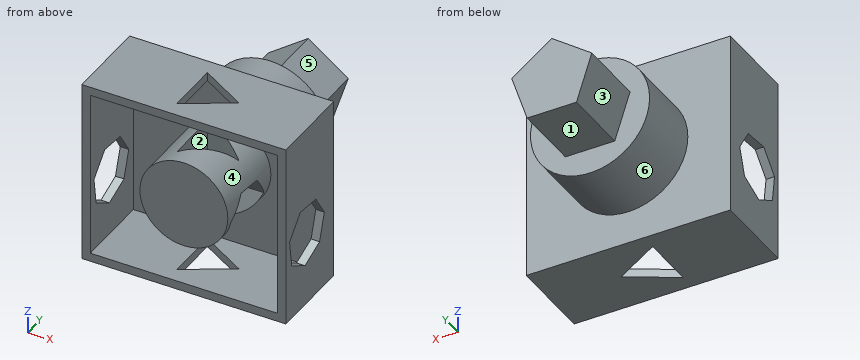
```python
from build123d import *

# Parameters (mm, degrees)
F0_W      = 76.2
F0_H      = 68.939676
F10_DEPTH = 31.75
F1_T      = -3.175
F2_R      = 22.225
F3_DEPTH  = 25.4
F5_DEPTH  = 25.4
F11_R     = 16.418379
F6_DEPTH  = 28.575
F8_DEPTH  = 76.201
F12_DEPTH = 68.940675


with BuildPart() as f10:
    # F0 (on Front) → F10 (new body)
    with BuildSketch(Plane.XZ):
        Rectangle(F0_W, F0_H)
    extrude(amount=F10_DEPTH)

    # F1
    f1_openings = [f10.faces().sort_by_distance(p)[0] for p in [
        (0, -31.75, 0),
    ]]
    offset(amount=F1_T, openings=f1_openings)

    # F2 (on face) → F3 (join)
    with BuildSketch(Plane(origin=(0, 0, 0), x_dir=(-1, 0, 0), z_dir=(0, 1, 0))):
        Circle(F2_R)
    extrude(amount=F3_DEPTH)

    # F4 (on face) → F5 (join)
    with BuildSketch(Plane(origin=(0, 25.4, 0), x_dir=(-1, 0, 0), z_dir=(0, 1, 0))):
        Polygon((-9.22709, -12.7), (9.22709, -12.7), (14.929745, 4.850968), (0, 15.698063), (-14.929745, 4.850968), align=None)
    extrude(amount=F5_DEPTH)

    # F11 (on face) → F6 (join, through all)
    with BuildSketch(Plane.XZ.offset(3.175)):
        Circle(F11_R)
    extrude(amount=F6_DEPTH)

    # F7 (on face) → F8 (cut, through all)
    with BuildSketch(Plane.YZ.offset(38.1)):
        Polygon((-27.926964, -13.740439), (-19.06612, -19.032735), (-9.40379, -15.40474), (-6.215907, -5.588409), (-11.903011, 3.024361), (-22.182597, 3.947978), (-29.313927, -3.51306), align=None)
    extrude(amount=-F8_DEPTH, mode=Mode.SUBTRACT)

    # F9 (on face) → F12 (cut, through all)
    with BuildSketch(Plane.XY.offset(34.469838)):
        Polygon((-5.835976, -5.766792), (-5.835976, -25.983208), (11.671953, -15.875), align=None)
    extrude(amount=-F12_DEPTH, mode=Mode.SUBTRACT)


solid = f10.part
```
Here's how the part is built. I have some questions about the finished solid (model axes, mm). Face numbers are marked on the shaded views. A direction names the side the tool comes from. Round coordinates to 2 decimals unless told otherwise and drop trailing zeros. Write each loop counter-clockwise with the first axis right and the second up, starting at its lowest first coordinate (ties: lowest second). Pieces come first, ordered by that corner, then holes.
Q1. If we section it at D-D on z = 9: Write out the boundary of the cut face in (x, y) (3 decimals), plus the area to 3 significant figures.
Q2. If we section it at A-A on z = -24: Write out the boundary of the cut face in (x, y) (3 decimals).
Q3. If we mould it in two halves opening along X, with no side actions, what happens to the marked faces 1, 2 and 3? For each: +X half, -X half, draft (parallel to the pull), parting line (faces both ways), or undercut.
Q4. If we section it at B-B on x = -28: Write out the boundary of the cut face in (y, z) (3 decimals).
Q5. Which directions (+Z, -Z, +X, -X, +Y, -Y) give clear straight access to the entire face, cutting with the end or side of a thin tool? Please do the marked faces 4, 5 and 6.
Q6. Will these pins go through, and if not, where does the flat tip stop? P1, Ø1.5, axis at y = 15.5, z = 21, coming from the +X side; P2, Ø5.5, axis at x = -1, y = 38, coming from the -Z side; P3, Ø4, axis at x = -12, z = 27.5, coming from the +Y side.
Q7. Please list where these lines run through material, in increasing order: probe 1 along Y at (x, z) = (-16, 25.5) (3 decimals); probe 2 along X at (y, z) = (12, -0.5); probe 3 along Z at (x, y) = (28.5, -26).
Q8. If we section it at C-C on y = 30.5: Write out the boundary of the cut face in (x, z), plus the area to 3 significant figures.
Answer below:
1. outline: (-38.1, -31.75) - (-34.925, -31.75) - (-34.925, -3.175) - (-13.732, -3.175) - (-13.732, -31.75) - (13.732, -31.75) - (13.732, -3.175) - (34.925, -3.175) - (34.925, -31.75) - (38.1, -31.75) - (38.1, 0) - (20.321, 0) - (20.321, 25.4) - (9.219, 25.4) - (9.219, 50.8) - (-9.219, 50.8) - (-9.219, 25.4) - (-20.321, 25.4) - (-20.321, 0) - (-38.1, 0) - close; hole (-5.836, -25.983) - (11.672, -15.875) - (-5.836, -5.767) - close
1. area: 2,530 mm2
2. outline: (-38.1, -31.75) - (-34.925, -31.75) - (-34.925, -3.175) - (34.925, -3.175) - (34.925, -31.75) - (38.1, -31.75) - (38.1, 0) - (-38.1, 0) - close
3. face 1: draft
3. face 2: undercut
3. face 3: -X half
4. outline: (-31.75, -34.47) - (0, -34.47) - (0, 34.47) - (-31.75, 34.47) - (-31.75, 31.295) - (-3.175, 31.295) - (-3.175, -31.295) - (-31.75, -31.295) - close
5. face 4: -Y
5. face 5: +Z, +X, +Y
5. face 6: +Y
6. P1: stops at x = 9.16
6. P2: stops at z = -12.7
6. P3: stops at y = 0
7. probe 1: y = -3.175 to 0
7. probe 2: x = -22.22 to 22.22
7. probe 3: z = -34.47 to -31.29, 31.29 to 34.47
8. outline: (-14.93, 4.85) - (-9.23, -12.7) - (9.23, -12.7) - (14.93, 4.85) - (0, 15.7) - close
8. area: 586 mm2
